from build123d import *

# Parameters (mm, degrees)
SKETCH164_W                    = 34.7
SKETCH164_H                    = 9.5
PAD087_DEPTH                   = 10.2
SKETCH165_W                    = 34.7
SKETCH165_H                    = 8
POCKET082_DEPTH                = 8.4
SKETCH166_W                    = 11.3
SKETCH166_H                    = 8
PAD088_DEPTH                   = 3.8
SKETCH167_R                    = 1.5
PAD089_DEPTH                   = 7.5
FILLET035_R                    = 0.5
SKETCH168_W                    = 8.8
SKETCH168_H                    = 6.75
POCKET083_DEPTH                = 3.81
SKETCH170_W                    = 1.25
SKETCH170_H                    = 4
POCKET084_DEPTH                = 1.25
PAD090_DEPTH                   = 2.56
SKETCH171_R                    = 1.9
PAD091_DEPTH                   = 5
SKETCH172_R                    = 1.05
POCKET085_DEPTH                = 2.56
SKETCH173_R                    = 0.75
POCKET086_DEPTH                = 5
SKETCH174_W                    = 1
SKETCH174_H                    = 9.5
POCKET087_DEPTH                = 0.3
SKETCH175_W                    = 1
SKETCH175_H                    = 10.2
POCKET088_DEPTH                = 0.3
FILLET036_R                    = 0.2
FILLET037_R                    = 0.2
SKETCH176_R                    = 2
PAD092_DEPTH                   = 2.8
FILLET038_R                    = 0.5
FILLET039_R                    = 0.5
SKETCH178_R                    = 1
PAD093_DEPTH                   = 1.1
FILLET040_R                    = 0.5
PAD162_DEPTH                   = 1
PART_MIRRORING_ROLL_ANGLE      = -90
PART_MIRRORING_PLACEMENT_ANGLE = -90


with BuildPart() as l_arm_shield:
    # Sketch164 → Pad087 (new body)
    with BuildSketch(Plane.XY):
        with Locations((-17.35, 0)):
            Rectangle(SKETCH164_W, SKETCH164_H)
    extrude(amount=PAD087_DEPTH)

    # Sketch165 (on Face6 of Pad087) → Pocket082 (cut)
    with BuildSketch(Plane.XY.offset(10.2)):
        with Locations((-17.35, 0.75)):
            Rectangle(SKETCH165_W, SKETCH165_H)
    extrude(amount=-POCKET082_DEPTH, mode=Mode.SUBTRACT)

    # Sketch166 (on Face6 of Pocket082) → Pad088 (join)
    with BuildSketch(Plane.XY.offset(1.8)):
        with Locations((-12.75, 0.75)):
            Rectangle(SKETCH166_W, SKETCH166_H)
    extrude(amount=PAD088_DEPTH)

    # Sketch167 (on Face6 of Pad088) → Pad089 (join)
    with BuildSketch(Plane.XY.offset(1.8)):
        with Locations((-22, 0.75)):
            Circle(SKETCH167_R)
    extrude(amount=PAD089_DEPTH)

    # Fillet035
    fillet035_edges = [l_arm_shield.edges().sort_by_distance(p)[0] for p in [
        (-17.35, -4.75, 0),
        (-34.7, -4.75, 5.1),
        (-34.7, 0, 0),
        (0, -4.75, 5.1),
        (0, 0, 0),
    ]]
    fillet(fillet035_edges, radius=FILLET035_R)

    # Sketch168 (on Face14 of Fillet035) → Pocket083 (cut)
    with BuildSketch(Plane.XY.offset(5.6)):
        with Locations((-12.75, 0.125)):
            Rectangle(SKETCH168_W, SKETCH168_H)
    extrude(amount=-POCKET083_DEPTH, mode=Mode.SUBTRACT)

    # Sketch170 (on Face13 of Pocket083) → Pocket084 (cut)
    with BuildSketch(Plane.XY.offset(5.6)):
        with Locations((-7.725, 0.75)):
            Rectangle(SKETCH170_W, SKETCH170_H)
    extrude(amount=-POCKET084_DEPTH, mode=Mode.SUBTRACT)

    # Sketch169 (on Face23 of Pocket083) → Pad090 (join)
    with BuildSketch(Plane.XY.offset(1.79)):
        with BuildLine():
            Line((-8.35, 2.75), (-11.5, 2.75))
            ThreePointArc((-11.5, 2.75), (-13.500002, 0.750015), (-11.500029, -1.25))
            Line((-11.500029, -1.25), (-8.35, -1.25))
            Line((-8.35, -1.25), (-8.35, 2.75))
        make_face()
    extrude(amount=PAD090_DEPTH)

    # Sketch171 (on Face16 of Pad090) → Pad091 (join)
    with BuildSketch(Plane.XY.offset(1.79)):
        with Locations((-15.5, 0.75)):
            Circle(SKETCH171_R)
    extrude(amount=PAD091_DEPTH)

    # Sketch172 (on Face26 of Pad091) → Pocket085 (cut)
    with BuildSketch(Plane.XY.offset(4.35)):
        with Locations((-11.5, 0.75)):
            Circle(SKETCH172_R)
    extrude(amount=-POCKET085_DEPTH, mode=Mode.SUBTRACT)

    # Sketch173 (on Face37 of Pocket085) → Pocket086 (cut)
    with BuildSketch(Plane.XY.offset(6.79)):
        with Locations((-15.5, 0.75)):
            Circle(SKETCH173_R)
    extrude(amount=-POCKET086_DEPTH, mode=Mode.SUBTRACT)

    # Sketch174 (on Face20 of Pocket086) → Pocket087 (cut)
    with BuildSketch(Plane(origin=(0, 0, 0), x_dir=(1, 0, 0), z_dir=(0, 0, -1))):
        with BuildLine():
            ThreePointArc((-27.95, 2.25), (-30.2, 0), (-27.95, -2.25))
            Line((-27.95, -2.25), (-11.95, -2.25))
            ThreePointArc((-11.95, -2.25), (-9.7, 0), (-11.95, 2.25))
            Line((-27.95, 2.25), (-11.95, 2.25))
        make_face()
        with Locations((-6.95, 0)):
            Rectangle(SKETCH174_W, SKETCH174_H)
    extrude(amount=-POCKET087_DEPTH, mode=Mode.SUBTRACT)

    # Sketch175 (on Face10 of Pocket087) → Pocket088 (cut)
    with BuildSketch(Plane.XZ.offset(4.75)):
        with Locations((-6.95, 5.1)):
            Rectangle(SKETCH175_W, SKETCH175_H)
    extrude(amount=-POCKET088_DEPTH, mode=Mode.SUBTRACT)

    # Fillet036
    fillet036_edges = [l_arm_shield.edges().sort_by_distance(p)[0] for p in [
        (-9.7, 0, 0),
        (-19.95, 2.25, 0),
        (-19.95, -2.25, 0),
        (-30.2, 0, 0),
    ]]
    fillet(fillet036_edges, radius=FILLET036_R)

    # Fillet037
    fillet037_edges = [l_arm_shield.edges().sort_by_distance(p)[0] for p in [
        (-7.45, 0.25, 0),
        (-6.45, 0.25, 0),
        (-7.45, -4.352155, 0.010547),
        (-7.45, -4.603553, 0.146447),
        (-7.45, -4.739453, 0.397845),
        (-7.45, -4.75, 5.35),
        (-6.45, -4.75, 5.35),
        (-6.45, -4.739453, 0.397845),
        (-6.45, -4.603553, 0.146447),
        (-6.45, -4.352155, 0.010547),
    ]]
    fillet(fillet037_edges, radius=FILLET037_R)

    # Sketch176 (on Face13 of Fillet037) → Pad092 (join)
    with BuildSketch(Plane.XZ.offset(4.75)):
        with Locations((-16.6, 5.1)):
            Circle(SKETCH176_R)
    extrude(amount=PAD092_DEPTH)

    # Fillet038
    fillet038_edges = [l_arm_shield.edges().sort_by_distance(p)[0] for p in [
        (-18.6, -7.55, 5.1),
    ]]
    fillet(fillet038_edges, radius=FILLET038_R)

    # Fillet039
    fillet039_edges = [l_arm_shield.edges().sort_by_distance(p)[0] for p in [
        (-7.1, 4.75, 3.7),
        (-18.4, 4.75, 3.7),
    ]]
    fillet(fillet039_edges, radius=FILLET039_R)

    # Sketch178 (on Face71 of Fillet039) → Pad093 (join)
    with BuildSketch(Plane.XZ.offset(7.55)):
        with Locations((-16.6, 5.1)):
            Circle(SKETCH178_R)
    extrude(amount=PAD093_DEPTH)

    # Fillet040
    fillet040_edges = [l_arm_shield.edges().sort_by_distance(p)[0] for p in [
        (-17.6, -8.65, 5.1),
    ]]
    fillet(fillet040_edges, radius=FILLET040_R)

    # Sketch283 (on Face11 of Fillet040) → Pad162 (join)
    with BuildSketch(Plane.XY.offset(10.2)):
        with BuildLine():
            Line((0, -3.25), (0, -4.25))
            ThreePointArc((-0.5, -4.75), (-0.146447, -4.603553), (0, -4.25))
            Line((-0.5, -4.75), (-6.25, -4.75))
            ThreePointArc((-6.45, -4.55), (-6.391421, -4.691421), (-6.25, -4.75))
            Line((-6.45, -4.55), (-6.45, -4.45))
            Line((-6.45, -4.45), (-7.45, -4.45))
            Line((-7.45, -4.45), (-7.45, -4.55))
            ThreePointArc((-7.65, -4.75), (-7.508579, -4.691421), (-7.45, -4.55))
            Line((-7.65, -4.75), (-34.2, -4.75))
            ThreePointArc((-34.7, -4.25), (-34.553553, -4.603553), (-34.2, -4.75))
            Line((-34.7, -4.25), (-34.7, -3.25))
            Line((-34.7, -3.25), (0, -3.25))
        make_face()
    extrude(amount=PAD162_DEPTH)


with BuildPart() as obj1:
    # Part__Mirroring: instance of L_Arm_Shield
    add(l_arm_shield.part.mirror(Plane(origin=(0, 0, 0), x_dir=(0, 1, 0), z_dir=(0, 0, 1))))


with BuildPart() as obj1_1:
    # Part__Mirroring roll: moved
    add(obj1.part.rotate(Axis((0, 0, 0), (1, 0, 0)), PART_MIRRORING_ROLL_ANGLE))


with BuildPart() as obj1_2:
    # Part__Mirroring placement: moved
    add(obj1_1.part.moved(Location((49.15, -55.7, 8))).rotate(Axis((49.15, -55.7, 8), (0, 0, 1)), PART_MIRRORING_PLACEMENT_ANGLE))


solid = obj1_2.part
The listing builds one solid part. Answer for the finished solid, in the listing's coordinates (mm). A direction names the side the tool comes from. Round coordinates to 2 decimals unless told otherwise and drop trailing zeros. Loops run counter-clockwise (first coordinate to the right, second up) from the corner with the lowest first, then second, coordinate; pieces in that order, holes last. Notation, with made-up numbers: M -23,13.5 L -8,13.5 A21 cw -8,44.5 Z; hole C 25.5,65 d6. An arc over 180 degrees is marked long. Return JSON: item names as keys, results as strings.
Q1. Find section D-D, the plane x = 39.5. Determine the outline of the cut face in (y, z).
Results list:
{"outline": "M -55.7,11.25 L -21,11.25 L -21,12.25 A0.5 ccw -21.5,12.75 L -48.05,12.75 A0.2 ccw -48.25,12.55 L -48.25,12.45 L -49.25,12.45 L -49.25,12.55 A0.2 ccw -49.45,12.75 L -55.2,12.75 A0.5 ccw -55.7,12.25 Z"}
Q2. The mould has two halves that part along Y. Classify faces 1 (the face through (49.15, -35, 11)), 2 (the face through (45, -37.3, 8)), 3 (the face through (44.816, -40.947, 13.884)): released by +Y, released by -Y, zero draft, split by the parting line, or undercut.
Results list:
{"face 1": "zero draft", "face 2": "undercut", "face 3": "split by the parting line"}
Q3. Which of the six approach directions +Z, -Z, +X, -X, +Y, -Y give full straight-line access (tool end or side, diameter ignored) to faces 4 (the face through (47.36, -42, 9)), 5 (the face through (47.35, -52, 7)), 6 (the face through (39.85, -34, 7)), 7 (the face through (44, -48, 5.25)), 8 (the face through (45.026, -38.883, 15.846))?
Results list:
{"face 4": "-X", "face 5": "-Z, -X, -Y", "face 6": "-Z, -X, +Y, -Y", "face 7": "-X, -Y", "face 8": "+Z"}
Q4. Find the intervals of material crossed by line 1 along Z through (x, y) = (46.5, -44.2); line 2 along Z through (x, y) = (43.75, -40.2); line 3 along Y through (x, z) = (45.5, 11), in increasing order. Write a range as from..to.
Results list:
{"line 1": "z = 3.25..4.5, 5.25..6.2, 8.3..9.25, 11.25..12.75", "line 2": "z = 3.25..4.5, 5.35..6.5, 8..9.15, 11.25..15.55", "line 3": "y = -48.6..-47.35, -38.55..-37.3"}
Q5. Each of these flat-tipped pins is pushed along its axis until it touches: pin 1 Ø2.5 at (y, z) = (-40.2, 7.25) entering from -X; pin 2 Ø1.4 at (x, z) = (46, 5.5) entering from -Y; pin 3 Ø2.5 at (y, z) = (-44.2, 7.25) entering from +X. Where does it stop, or does it pass through?
Results list:
{"pin 1": "stops at x = 42.36", "pin 2": "stops at y = -48.6", "pin 3": "stops at x = 48.85"}
Q6. Find section B-B, the plane x = 41. Determine the outline of the cut face in (y, z).
Results list:
{"outline": "M -55.7,11.25 L -21,11.25 L -21,12.25 A0.5 ccw -21.5,12.75 L -48.05,12.75 A0.2 ccw -48.25,12.55 L -48.25,12.45 L -49.25,12.45 L -49.25,12.55 A0.2 ccw -49.45,12.75 L -55.2,12.75 A0.5 ccw -55.7,12.25 Z; C -33.7,7.25 d3"}
Q7. Find section A-A, the plane y = -33.7. Determine the outline of the cut face in (x, z).
Results list:
{"outline": "M 37.95,11.25 L 47.35,11.25 L 47.35,8.75 L 39.85,8.75 L 39.85,5.75 L 47.35,5.75 L 47.35,3.25 L 49.15,3.25 L 49.15,5.55 A0.2 ccw 48.95,5.75 L 48.85,5.75 L 48.85,10.25 L 48.95,10.25 A0.2 ccw 49.15,10.45 L 49.15,12.25 A0.5 ccw 48.65,12.75 L 37.95,12.75 Z"}
Q8. Find section C-C, the plane x = 44.05. State how many separate pieces and enclosed holes the cut face has, plus the area to 3 significant figures.
Results list:
{"separate pieces": "2", "enclosed holes": "1", "area": "107 mm2"}
